The drawing under review shows one solid part. Ordinate dimensions are in mm from its lowest x, y, z. A direction names the side the tool comes from. Coordinates: 2 decimals unless noted, no trailing zeros. Write each loop counter-clockwise with the first axis right and the second up, starting at its lowest first coordinate (ties: lowest second). Pieces come first, ordered by that corner, then holes. Notation, with made-up numbers: (51.5, 79) -> (91.5, 79) arc R23 cw to (91.5, 104) -> close; hole circle Ø5 at (-38, 2). An arc over 180 degrees is marked (long way). One line per item, written item: value. Start each with the question number.
1) Add section C-C (z = 4.25). State the section outline as (x, y) points.
2) Add section D-D (y = 10.75). State the section outline as (x, z) points, and give its area (3 significant figures).
3) For pin 1 Ø1.6 at (x, y) = (7, 12) entering from +Z, flat-tipped, find the tip position at first contact; note if it passes through.
4) Machinability: for the marked faces 1 and 2, which of the approach directions +Z, -Z, +X, -X, +Y, -Y give a long, thin tool a straight path to every point of the face, cutting with its end or side? Answer none if there is none.
5) Mouldability with a two-part tool opening along X and no side actions: class the marked faces 3, 4 and 5 as released by +X, released by -X, zero draft, split by the parting line, or undercut.
6) For probe 1 along Y at (x, z) = (5, 20.5); probe 2 along X at (y, z) = (4, 19.25); probe 3 along Z at (x, y) = (8, 12.75), list the stretches that pass through material, from the lowest coordinate up. Write a range as from..to.
7) Add section B-B (z = 16.5). State the section outline as (x, y) points.
8) Add section A-A (x = 0.5). State the section outline as (y, z) points, and give its area (4 significant figures).
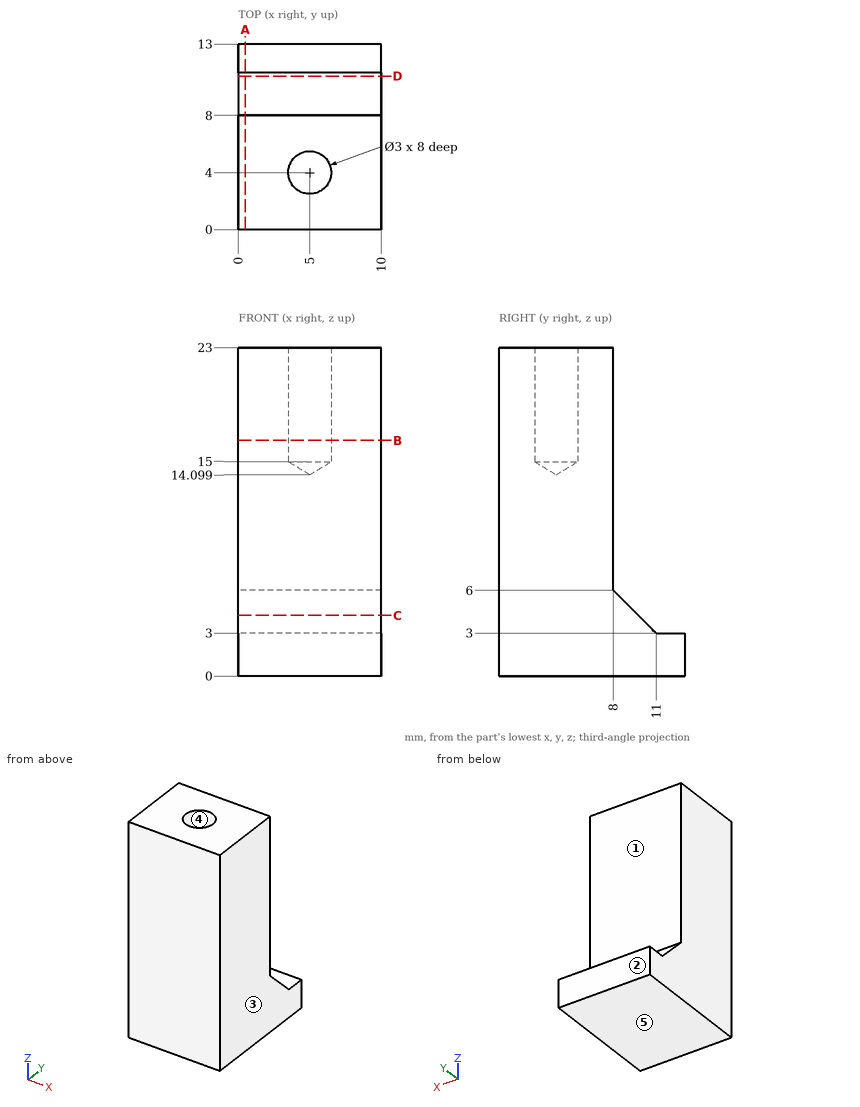
Numbers:
1. outline: (0, 0) -> (10, 0) -> (10, 9.75) -> (0, 9.75) -> close
2. outline: (0, 0) -> (10, 0) -> (10, 3.25) -> (0, 3.25) -> close
2. area: 32.5 mm²
3. pin 1: z = 3
4. face 1: +Z, +X, -X, +Y
4. face 2: +Z, -Z, +X, -X, +Y
5. face 3: released by +X
5. face 4: undercut
5. face 5: zero draft
6. probe 1: 0..2.5, 5.5..8
6. probe 2: 0..3.5, 6.5..10
6. probe 3: 0..3
7. outline: (0, 0) -> (10, 0) -> (10, 8) -> (0, 8) -> close; hole circle Ø3 at (5, 4)
8. outline: (0, 0) -> (13, 0) -> (13, 3) -> (11, 3) -> (8, 6) -> (8, 23) -> (0, 23) -> close
8. area: 203.5 mm²
